Autodesk Inventor part; units mm, degrees
ref_plane "YZ Plane" through (0, 0, 0) normal (1, 0, 0) x (0, 1, 0)
ref_plane "XZ Plane" through (0, 0, 0) normal (0, 1, 0) x (-1, 0, 0)
ref_plane "XY Plane" through (0, 0, 0) normal (0, 0, 1) x (1, 0, 0)
sketch "スケッチ1" plane through (0, 0, 0) normal (1, 0, 0) x (0, 1, 0)
  line L0 (-4.5, 0) -> (4.5, 0)
  line L1 (0, 0) -> (0, 3.1754) construction
  line L2 (-4.2544, 3.1754) -> (-4.5, 2.75)
  line L3 (-4.5, 2.75) -> (-4.5, 0)
  line L4 (-4.2544, 3.1754) -> (4.2544, 3.1754)
  line L5 (4.2544, 3.1754) -> (4.5, 2.75)
  line L6 (4.5, 2.75) -> (4.5, 0)
  dimension "d1" = 2.75
  dimension "d2" = 3.1754
  dimension "d3" = 30
  dimension "d4" = 9
revolve "回転1" add sketch "スケッチ1" angle 360 about axis through (0, -4.5, 0) along (0, 1, 0)
sketch "スケッチ2" plane through (0, 4.5, 0) normal (0, 1, 0) x (1, 0, 0)
  circle A0 centre (0, 0) radius 3.1754
  line L0 (1.5877, 2.75) -> (3.1754, 0)
  line L1 (3.1754, 0) -> (1.5877, -2.75)
  line L2 (1.5877, -2.75) -> (-1.5877, -2.75)
  line L3 (-1.5877, -2.75) -> (-3.1754, 0)
  line L4 (-3.1754, 0) -> (-1.5877, 2.75)
  line L5 (-1.5877, 2.75) -> (1.5877, 2.75)
  point P0 (0, 0)
  point P1 (-1.5877, 2.75)
  point P2 (-1.5877, 2.75)
  point P3 (-3.1754, 0)
  point P4 (-3.1754, 0)
  point P5 (1.5877, -2.75)
  point P6 (1.5877, -2.75)
  point P7 (3.1754, 0)
  point P8 (3.1754, 0)
extrude "押し出し1" cut sketch "スケッチ2" against normal through all contours L0 A0 | A0 L1 | L5 A0 | A0 L2 | L4 A0 | A0 L3
hole "穴1" at (0, 4.5, 0) direction (0, -1, 0) diameter 2.459 end through all countersink diameter 3 countersink angle 90
mirror "ミラー1" about plane through (0, 0, 0) normal (0, 1, 0) of "穴1"
equation "\"d2\" = 1.1547 * d1"
properties part number "ASL-309BE" material "アルミニウム 2014-T4"
Input: part model. Units: mm. Frame: model coordinates. Give positions to 0.01 mm unless a question says otherwise; leave off trailing zeros. Loops run counter-clockwise (first coordinate to the right, second up) from the corner with the lowest first, then second, coordinate; pieces in that order, holes last. Notation, with made-up numbers: (71, 6) - (92, 6) arc R16 ccw to (92, 13) - close; hole circle Ø10 at (-22.75, 70.25). An arc over 180 degrees is marked (long way). Use CSV: the item, a comma, the result in double quotes. Start each with the question number.
Item 1: Contact query for a flat-ended pin moving along its axis: P1, Ø1.5, axis at y = 2, z = 1.5, coming from the -X side. Output: stop coordinate, or through.
Item 2: Section A-A on y = -3. Return loops of the section in (x, z).
Item 3: Line query: line 1 (Z direction, x = 0, y = -1.75); line 2 (Z direction, x = -0.5, y = -3); line 3 (X direction, y = 2, z = 0.7). Output: solid intervals per line, ascending.
Item 4: Mould query, pull axis Z, two halves, no side actions, for faces 1 (the cylindrical face through (0.748, -0.059, -0.976)), 2 (the flat face through (-1.2, 4.5, 1.2)), 3 (the conical face through (1.44, -4.41, 2.52)), 4 (the conical face through (1.44, 4.41, -2.52)). Classes: pulls with the +Z half, pulls with the -Z half, needs draft (parallel to the pull), parting line crosses it, or undercut.
Ans:
1,P1,"stops at x = -2.74"
2,outline,"(-3.18, 0) - (-1.59, -2.75) - (1.59, -2.75) - (3.18, 0) - (1.59, 2.75) - (-1.59, 2.75) - close; hole circle Ø2.46 at (0, 0)"
3,line 1,"z = -2.75 to -1.23, 1.23 to 2.75"
3,line 2,"z = -2.75 to -1.12, 1.12 to 2.75"
3,line 3,"x = -2.77 to -1.01, 1.01 to 2.77"
4,face 1,"undercut"
4,face 2,"needs draft"
4,face 3,"pulls with the +Z half"
4,face 4,"pulls with the -Z half"
